Autodesk Inventor part; units mm, degrees
ref_plane "YZ Plane" through (0, 0, 0) normal (1, 0, 0) x (0, 1, 0)
ref_plane "XZ Plane" through (0, 0, 0) normal (0, 1, 0) x (-1, 0, 0)
ref_plane "XY Plane" through (0, 0, 0) normal (0, 0, 1) x (1, 0, 0)
sketch "Эскиз1" plane through (0, 0, 0) normal (0, 0, 1) x (1, 0, 0)
  line L0 (-60, 0) -> (60, 0)
  line L1 (60, 0) -> (41.2436, 70)
  line L2 (41.2436, 70) -> (-41.2436, 70)
  line L3 (-41.2436, 70) -> (-60, 0)
  line L4 (0, 70) -> (0, 0)
  line L5 (-57.3935, 2) -> (-39.7089, 68)
  line L6 (-39.7089, 68) -> (39.7089, 68)
  line L7 (39.7089, 68) -> (57.3935, 2)
  line L8 (57.3935, 2) -> (-57.3935, 2)
  dimension "d0" = 70
  dimension "d1" = 120
  dimension "d2" = 75
  dimension "d8" = 2
  dimension "d9" = 2
  dimension "d10" = 2
  dimension "d11" = 2
  dimension "d12" = 0
extrude "Выдавливание1" add sketch "Эскиз1" along normal blind 120 contours L3 L2 L4 L6 L5 L8 L0 | L4 L8 L7 L6 L2 L1 L0
sketch "Эскиз2" plane through (0, 0, 0) normal (1, 0, 0) x (0, 1, 0)
  line L0 (0, 0) -> (0, 120)
  line L1 (0, 0) -> (70, 18.7564)
  line L2 (70, 0) -> (70, 120)
  line L3 (70, 18.7564) -> (70, 101.2436)
  line L4 (70, 0) -> (70, 120)
  line L5 (70, 120) -> (0, 120)
  line L6 (70, 101.2436) -> (0, 120)
  line L7 (0, 120) -> (0, 0)
  line L8 (70, 60) -> (0, 60)
  dimension "d5" = 75
extrude "Выдавливание2" cut sketch "Эскиз2" along normal mid plane 1000 contours L0 L8 L2 L1 | L0 L6 L2 L8 keep common part
sketch "Эскиз3" plane through (0, 0, 0) normal (1, 0, 0) x (0, 1, 0)
  line L0 (0, 0) -> (0, 120)
  line L1 (70, 18.7564) -> (70, 101.2436)
  line L2 (0, 0) -> (70, 18.7564)
  line L3 (70, 18.7564) -> (70, 20.7564)
  line L4 (70, 20.7564) -> (0, 2)
  line L5 (70, 18.7564) -> (0, 0)
  line L6 (0, 2) -> (0, 0)
  line L7 (0, 120) -> (70, 101.2436)
  line L8 (68, 101.7795) -> (2, 119.4641)
  line L9 (70, 101.2436) -> (70, 99.2436)
  line L10 (70, 99.2436) -> (0, 118)
  line L11 (0, 120) -> (0, 118)
  point P0 (0, 2)
  dimension "d13" = 2
  dimension "d14" = 2
extrude "Выдавливание3" add sketch "Эскиз3" along normal mid plane 120 contours L0 L4 L1 L2 | L0 L7 L1 L10
sketch "Эскиз4" plane through (0, 0, 0) normal (0, 0, 1) x (1, 0, 0)
  line L0 (60, 70) -> (60, 0)
  line L1 (60, 0) -> (41.2436, 70)
  line L2 (60, 70) -> (-60, 70)
  line L3 (-41.2436, 70) -> (-60, 0)
  line L4 (41.2436, 70) -> (-41.2436, 70)
  line L5 (-41.2436, 70) -> (-60, 0)
  line L6 (-60, 0) -> (60, 0)
  line L7 (-60, 0) -> (60, 0)
  line L8 (60, 0) -> (41.2436, 70)
  point P0 (0, 0)
  dimension "d19" = 0
extrude "Выдавливание4" cut sketch "Эскиз4" along normal blind 120 contours L6 L3 L2 L1 keep common part
Verification items for the finished model (mm, model axes). A direction names the side the tool comes from. Round coordinates to 2 decimals unless told otherwise and drop trailing zeros. Order: outer loops, then holes, each group sorted by start corner. A loop starts at its lowest first (then second) coordinate and runs counter-clockwise, first axis right, second up. Notation, with made-up numbers: (61.5, -22.5) -> (100.5, -22.5) arc R19 cw to (100.5, -17.5) -> close; hole circle Ø11 at (8.5, 72.5). An arc over 180 degrees is marked (long way). Put each result on its own line as item: value.
1) Section check B-B (z = 83). Record the cut outline in (x, y), then the cut area to 3 significant figures.
Final values:
outline: (-60, 0) -> (60, 0) -> (41.24, 70) -> (-41.24, 70) -> close; hole (-57.39, 2) -> (57.39, 2) -> (39.71, 68) -> (-39.71, 68) -> close
area: 678 mm^2
2) Mould release check, pull along Z, two halves, no side actions. Record for faces 1 (the flat face through (-0.8, 35.46, 11.5)), 2 (the flat face through (-1, 0, 59)), 3 (the flat face through (-0.84, 34.51, 9.247)): +Z half, -Z half, draft (parallel to the pull), parting line (faces both ways), or undercut.
Final values:
face 1: undercut
face 2: draft
face 3: -Z half
3) Section check A-A (x = -25.5). Record the cut outline in (y, z), then the cut area to 3 significant figures.
Final values:
outline: (0, 0) -> (70, 18.76) -> (70, 101.24) -> (0, 120) -> close; hole (2, 2.54) -> (68, 20.22) -> (68, 99.78) -> (2, 117.46) -> close
area: 669 mm^2
4) Material ranges on line 1 (Y direction, x = 25, z = 21.5); line 2 (X direction, y = 47.5, z = 24); line 3 (X direction, y = 45, z = 40), recorded low to high.
Final values:
line 1: y = 0 to 2, 68 to 70
line 2: x = -47.27 to -45.2, 45.2 to 47.27
line 3: x = -47.94 to -45.87, 45.87 to 47.94
5) Section check C-C (y = 50.5). Record the cut outline in (x, z), then the cut area to 3 significant figures.
Final values:
outline: (-46.47, 13.53) -> (46.47, 13.53) -> (46.47, 106.47) -> (-46.47, 106.47) -> close; hole (-44.4, 15.53) -> (44.4, 15.53) -> (44.4, 104.47) -> (-44.4, 104.47) -> close
area: 740 mm^2
6) Set-up check for faces 4 (the flat face through (1, 70, 59)), 5 (the flat face through (-48.675, 34.538, 59.196)): record each of +Z, -Z, +X, -X, +Y, -Y from which the full face is reachable in a straight line by a thin tool's end or side.
Final values:
face 4: +Z, -Z, +X, -X, +Y
face 5: none
7) Depth check by flat-ended pin: pin 1 (1.5 mm diameter, centred on y = 33.5, z = 40.5, fed in from +X); pin 2 (24 mm diameter, centred on x = -6.5, z = 75, fed in from -Y); pin 3 (8 mm diameter, centred on x = -7.5, y = 40, fed in from -Z); pin 4 (4 mm diameter, centred on y = 30, z = 45, fed in from -X). Enter the tip coordinate at first touch or a pass-through.
Final values:
pin 1: stops at x = 51.22
pin 2: stops at y = 0
pin 3: stops at z = 9.65
pin 4: stops at x = -52.5
